```python
from build123d import *

# Parameters (mm, degrees)
SKETCH1_R      = 2.552699952
EXTRUDE1_DEPTH = 25.4


with BuildPart() as part:
    # Sketch1 → Extrude1 (new body)
    with BuildSketch(Plane.XY):
        with BuildLine():
            Line((-8.483605576, 7.293893252), (-5.545081932, 4.355385482))
            ThreePointArc((-5.545081932, 4.355385482), (-4.614735711, 3.132038282), (-4.177987221, 1.658480269))
            Line((-4.177987221, 1.658480269), (-4.177987221, -1.658480269))
            ThreePointArc((-4.177987221, -1.658480269), (-4.614735711, -3.132038282), (-5.545081932, -4.355385482))
            Line((-5.545081932, -4.355385482), (-8.483605576, -7.293893252))
            ThreePointArc((-8.483605576, -7.293893252), (-9.464416196, -7.488986523), (-10.019999931, -6.657495349))
            Line((-10.019999931, -6.657495349), (-10.019999685, -4.25451262))
            ThreePointArc((-10.019999685, -4.25451262), (-10.317579227, -3.536092054), (-11.035999792, -3.238512512))
            Line((-11.035999792, -3.238512512), (-11.226349864, -3.237859075))
            ThreePointArc((-11.226349864, -3.237859075), (-11.933208752, -3.520692129), (-12.24510272, -4.215217994))
            Line((-12.24510272, -4.215217994), (-12.499999765, -10.913485754))
            ThreePointArc((-12.499999765, -10.913485754), (-12.014686132, -12.056001152), (-10.855475092, -12.4999612))
            Line((-10.855475092, -12.4999612), (-4.22175692, -12.26151704))
            ThreePointArc((-4.22175692, -12.26151704), (-3.524602107, -11.952788933), (-3.238512512, -11.246042429))
            Line((-3.238512512, -11.246042429), (-3.238512512, -11.035999792))
            ThreePointArc((-3.238512512, -11.035999792), (-3.536092054, -10.317579227), (-4.25451262, -10.019999685))
            Line((-4.25451262, -10.019999685), (-6.657495349, -10.019999931))
            ThreePointArc((-6.657495349, -10.019999931), (-7.488986523, -9.464416196), (-7.293893252, -8.483605576))
            Line((-7.293893252, -8.483605576), (-4.355385482, -5.545081932))
            ThreePointArc((-4.355385482, -5.545081932), (-3.132038282, -4.614735711), (-1.658480269, -4.177987221))
            Line((-1.658480269, -4.177987221), (1.658480269, -4.177987221))
            ThreePointArc((1.658480269, -4.177987221), (3.132038282, -4.614735711), (4.355385482, -5.545081932))
            Line((4.355385482, -5.545081932), (7.293893252, -8.483605576))
            ThreePointArc((7.293893252, -8.483605576), (7.488986523, -9.464416196), (6.657495349, -10.019999931))
            Line((6.657495349, -10.019999931), (4.25451262, -10.019999685))
            ThreePointArc((4.25451262, -10.019999685), (3.536092054, -10.317579227), (3.238512512, -11.035999792))
            Line((3.238512512, -11.035999792), (3.238512512, -11.246042429))
            ThreePointArc((3.238512512, -11.246042429), (3.524602107, -11.952788933), (4.22175692, -12.26151704))
            Line((4.22175692, -12.26151704), (10.855475092, -12.4999612))
            ThreePointArc((10.855475092, -12.4999612), (12.014686132, -12.056001152), (12.499999765, -10.913485754))
            Line((12.499999765, -10.913485754), (12.24510272, -4.215217994))
            ThreePointArc((12.24510272, -4.215217994), (11.933208752, -3.520692129), (11.226349864, -3.237859075))
            Line((11.226349864, -3.237859075), (11.035999792, -3.238512512))
            ThreePointArc((11.035999792, -3.238512512), (10.317579227, -3.536092054), (10.019999685, -4.25451262))
            Line((10.019999685, -4.25451262), (10.019999931, -6.657495349))
            ThreePointArc((10.019999931, -6.657495349), (9.464416196, -7.488986523), (8.483605576, -7.293893252))
            Line((8.483605576, -7.293893252), (5.545081932, -4.355385482))
            ThreePointArc((5.545081932, -4.355385482), (4.614735711, -3.132038282), (4.177987221, -1.658480269))
            Line((4.177987221, -1.658480269), (4.177987221, 1.658480269))
            ThreePointArc((4.177987221, 1.658480269), (4.614735711, 3.132038282), (5.545081932, 4.355385482))
            Line((5.545081932, 4.355385482), (8.483605576, 7.293893252))
            ThreePointArc((8.483605576, 7.293893252), (9.464416196, 7.488986523), (10.019999931, 6.657495349))
            Line((10.019999931, 6.657495349), (10.019999685, 4.25451262))
            ThreePointArc((10.019999685, 4.25451262), (10.317579227, 3.536092054), (11.035999792, 3.238512512))
            Line((11.035999792, 3.238512512), (11.258353132, 3.237749214))
            ThreePointArc((11.258353132, 3.237749214), (11.966958292, 3.522261588), (12.277278698, 4.219950495))
            Line((12.277278698, 4.219950495), (12.499999765, 10.912499795))
            Line((12.499999765, 10.912499795), (12.499999765, 14.087499735))
            Line((12.499999765, 14.087499735), (12.277278698, 20.780049035))
            ThreePointArc((12.277278698, 20.780049035), (11.966958292, 21.477737942), (11.258353132, 21.762250316))
            Line((11.258353132, 21.762250316), (11.035999792, 21.761487018))
            ThreePointArc((11.035999792, 21.761487018), (10.317579227, 21.463907476), (10.019999685, 20.74548691))
            Line((10.019999685, 20.74548691), (10.019999931, 18.34250418))
            ThreePointArc((10.019999931, 18.34250418), (9.464416196, 17.511013007), (8.483605576, 17.706106278))
            Line((8.483605576, 17.706106278), (5.545081932, 20.644614048))
            ThreePointArc((5.545081932, 20.644614048), (4.614735711, 21.867961248), (4.177987221, 23.341519261))
            Line((4.177987221, 23.341519261), (4.177987221, 26.658479799))
            ThreePointArc((4.177987221, 26.658479799), (4.614735711, 28.132037812), (5.545081932, 29.355385011))
            Line((5.545081932, 29.355385011), (8.483605576, 32.293892782))
            ThreePointArc((8.483605576, 32.293892782), (9.464416196, 32.488986052), (10.019999931, 31.657494879))
            Line((10.019999931, 31.657494879), (10.019999685, 29.25451215))
            ThreePointArc((10.019999685, 29.25451215), (10.317579227, 28.536091584), (11.035999792, 28.238512042))
            Line((11.035999792, 28.238512042), (11.226349864, 28.237858605))
            ThreePointArc((11.226349864, 28.237858605), (11.933208752, 28.520691659), (12.24510272, 29.215217524))
            Line((12.24510272, 29.215217524), (12.499999765, 35.913485284))
            ThreePointArc((12.499999765, 35.913485284), (12.014686132, 37.056000682), (10.855475092, 37.499960729))
            Line((10.855475092, 37.499960729), (4.22175692, 37.261516569))
            ThreePointArc((4.22175692, 37.261516569), (3.524602107, 36.952788463), (3.238512512, 36.246041959))
            Line((3.238512512, 36.246041959), (3.238512512, 36.035999322))
            ThreePointArc((3.238512512, 36.035999322), (3.536092054, 35.317578756), (4.25451262, 35.019999214))
            Line((4.25451262, 35.019999214), (6.657495349, 35.019999461))
            ThreePointArc((6.657495349, 35.019999461), (7.488986523, 34.464415726), (7.293893252, 33.483605106))
            Line((7.293893252, 33.483605106), (4.355385482, 30.545081462))
            ThreePointArc((4.355385482, 30.545081462), (3.132038282, 29.614735241), (1.658480269, 29.177986751))
            Line((1.658480269, 29.177986751), (-1.658480269, 29.177986751))
            ThreePointArc((-1.658480269, 29.177986751), (-3.132038282, 29.614735241), (-4.355385482, 30.545081462))
            Line((-4.355385482, 30.545081462), (-7.293893252, 33.483605106))
            ThreePointArc((-7.293893252, 33.483605106), (-7.488986523, 34.464415726), (-6.657495349, 35.019999461))
            Line((-6.657495349, 35.019999461), (-4.25451262, 35.019999214))
            ThreePointArc((-4.25451262, 35.019999214), (-3.536092054, 35.317578756), (-3.238512512, 36.035999322))
            Line((-3.238512512, 36.035999322), (-3.238512512, 36.246041959))
            ThreePointArc((-3.238512512, 36.246041959), (-3.524602107, 36.952788463), (-4.22175692, 37.261516569))
            Line((-4.22175692, 37.261516569), (-10.855475092, 37.499960729))
            ThreePointArc((-10.855475092, 37.499960729), (-12.014686132, 37.056000682), (-12.499999765, 35.913485284))
            Line((-12.499999765, 35.913485284), (-12.24510272, 29.215217524))
            ThreePointArc((-12.24510272, 29.215217524), (-11.933208752, 28.520691659), (-11.226349864, 28.237858605))
            Line((-11.226349864, 28.237858605), (-11.035999792, 28.238512042))
            ThreePointArc((-11.035999792, 28.238512042), (-10.317579227, 28.536091584), (-10.019999685, 29.25451215))
            Line((-10.019999685, 29.25451215), (-10.019999931, 31.657494879))
            ThreePointArc((-10.019999931, 31.657494879), (-9.464416196, 32.488986052), (-8.483605576, 32.293892782))
            Line((-8.483605576, 32.293892782), (-5.545081932, 29.355385011))
            ThreePointArc((-5.545081932, 29.355385011), (-4.614735711, 28.132037812), (-4.177987221, 26.658479799))
            Line((-4.177987221, 26.658479799), (-4.177987221, 23.341519261))
            ThreePointArc((-4.177987221, 23.341519261), (-4.614735711, 21.867961248), (-5.545081932, 20.644614048))
            Line((-5.545081932, 20.644614048), (-8.483605576, 17.706106278))
            ThreePointArc((-8.483605576, 17.706106278), (-9.464416196, 17.511013007), (-10.019999931, 18.34250418))
            Line((-10.019999931, 18.34250418), (-10.019999685, 20.74548691))
            ThreePointArc((-10.019999685, 20.74548691), (-10.317579227, 21.463907476), (-11.035999792, 21.761487018))
            Line((-11.035999792, 21.761487018), (-11.258353132, 21.762250316))
            ThreePointArc((-11.258353132, 21.762250316), (-11.966958292, 21.477737942), (-12.277278698, 20.780049035))
            Line((-12.277278698, 20.780049035), (-12.499999765, 14.087499735))
            Line((-12.499999765, 14.087499735), (-12.499999765, 10.912499795))
            Line((-12.499999765, 10.912499795), (-12.277278698, 4.219950495))
            ThreePointArc((-12.277278698, 4.219950495), (-11.966958292, 3.522261588), (-11.258353132, 3.237749214))
            Line((-11.258353132, 3.237749214), (-11.035999792, 3.238512512))
            ThreePointArc((-11.035999792, 3.238512512), (-10.317579227, 3.536092054), (-10.019999685, 4.25451262))
            Line((-10.019999685, 4.25451262), (-10.019999931, 6.657495349))
            ThreePointArc((-10.019999931, 6.657495349), (-9.464416196, 7.488986523), (-8.483605576, 7.293893252))
        make_face()
        Circle(SKETCH1_R, mode=Mode.SUBTRACT)
        with Locations((0, 24.99999953)):
            Circle(SKETCH1_R, mode=Mode.SUBTRACT)
        with BuildLine():
            Line((-4.532162174, 5.36830524), (-7.449420439, 8.285579265))
            ThreePointArc((-7.449420439, 8.285579265), (-8.351141741, 8.889360855), (-9.418419027, 9.085760214))
            ThreePointArc((-9.418419027, 9.085760214), (-10.5176918, 9.519951543), (-10.975999794, 10.60939017))
            Line((-10.975999794, 10.60939017), (-10.975999794, 14.39060936))
            ThreePointArc((-10.975999794, 14.39060936), (-10.5176918, 15.480047987), (-9.418419027, 15.914239316))
            ThreePointArc((-9.418419027, 15.914239316), (-8.351141741, 16.110638675), (-7.449420439, 16.714420265))
            Line((-7.449420439, 16.714420265), (-4.532162174, 19.63169429))
            ThreePointArc((-4.532162174, 19.63169429), (-3.213705709, 20.512658734), (-1.658480269, 20.822012308))
            Line((-1.658480269, 20.822012308), (1.658480269, 20.822012308))
            ThreePointArc((1.658480269, 20.822012308), (3.213705709, 20.512658734), (4.532162174, 19.63169429))
            Line((4.532162174, 19.63169429), (7.449420439, 16.714420265))
            ThreePointArc((7.449420439, 16.714420265), (8.351141741, 16.110638675), (9.418419027, 15.914239316))
            ThreePointArc((9.418419027, 15.914239316), (10.5176918, 15.480047987), (10.975999794, 14.39060936))
            Line((10.975999794, 14.39060936), (10.975999794, 10.60939017))
            ThreePointArc((10.975999794, 10.60939017), (10.5176918, 9.519951543), (9.418419027, 9.085760214))
            ThreePointArc((9.418419027, 9.085760214), (8.351141741, 8.889360855), (7.449420439, 8.285579265))
            Line((7.449420439, 8.285579265), (4.532162174, 5.36830524))
            ThreePointArc((4.532162174, 5.36830524), (3.213705709, 4.487340795), (1.658480269, 4.177987221))
            Line((1.658480269, 4.177987221), (-1.658480269, 4.177987221))
            ThreePointArc((-1.658480269, 4.177987221), (-3.213705709, 4.487340795), (-4.532162174, 5.36830524))
        make_face(mode=Mode.SUBTRACT)
    extrude(amount=EXTRUDE1_DEPTH)


solid = part.part
```
Build history of the part. All positions in model axes, mm. A direction names the side the tool comes from. Give positions to 0.01 mm unless a question says otherwise; leave off trailing zeros. Loops run counter-clockwise (first coordinate to the right, second up) from the corner with the lowest first, then second, coordinate; pieces in that order, holes last.
1) 3-axis set-ups, long thin cutter, end or side, ignore diameter. For faces 1 (the face through (0, -4.178, 13)), 2 (the face through (-5.845, -7.035, 12.522)): which of +Z, -Z, +X, -X, +Y, -Y reach the whole face in a straight line?
Values follow:
face 1: +Z, -Z, -Y
face 2: +Z, -Z
2) Band-saw the part on C-C on z = 5.5. State how many separate pieces and enclosed holes the cut face has, then the cut area to 3 significant figures.
Values follow:
separate pieces: 1
enclosed holes: 3
area: 434 mm2
3) Drop flat-ended pins along their axis: P1, Ø1.5, axis at x = 7.5, y = 15, coming from the +Z side; P2, Ø1.2, axis at y = 30.5, z = 16.5, coming from the -X side; P3, Ø0.7, axis at x = 5.5, z = 11, coming from the +Y side; P4, Ø3.5, axis at x = 0, z = 17.5, coming from the +Y side. Give the stop position or say it passes through.
Values follow:
P1: passes through
P2: stops at x = -12.32
P3: stops at y = 37.32
P4: stops at y = 29.19
4) Band-saw the part on B-B on y = 25. List the corners of the cut face in (x, z), then the cut area to 3 significant figures.
Values follow:
outline: (-4.18, 0) - (-2.55, 0) - (-2.55, 25.4) - (-4.18, 25.4) - close; (2.55, 0) - (4.18, 0) - (4.18, 25.4) - (2.55, 25.4) - close
area: 82.6 mm2
5) Band-saw the part on A-A on x = 0. List the corners of the cut face in (y, z).
Values follow:
outline: (-4.18, 0) - (-2.55, 0) - (-2.55, 25.4) - (-4.18, 25.4) - close; (2.55, 0) - (4.18, 0) - (4.18, 25.4) - (2.55, 25.4) - close; (20.82, 0) - (22.45, 0) - (22.45, 25.4) - (20.82, 25.4) - close; (27.55, 0) - (29.18, 0) - (29.18, 25.4) - (27.55, 25.4) - close
6) Two-plate mould, pull along X, no slides. Class faces 3 (the face through (-10.51, 9.51, 12.52)), 4 (the face through (12.374, -7.611, 12.522)), 5 (the face through (-4.178, 0, 13)): released by +X, released by -X, zero draft, split by the parting line, or undercut.
Values follow:
face 3: undercut
face 4: released by +X
face 5: released by -X
7) Probe line 1 along Y through (x, z) = (0, 20); line 2 along X through (y, z) = (31.5, 11.75); line 3 along X through (y, z) = (21, 3.5). List the from-to ranges inside material, lowest first.
Values follow:
line 1: y = -4.18 to -2.55, 2.55 to 4.18, 20.82 to 22.45, 27.55 to 29.18
line 2: x = -12.33 to -10.02, -7.69 to -5.31, 5.31 to 7.69, 10.02 to 12.33
line 3: x = -12.25 to -10.05, -5.2 to 5.2, 10.05 to 12.25
